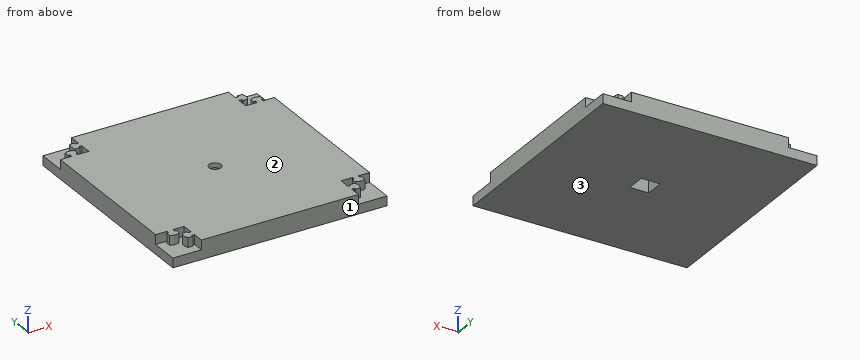
```python
from build123d import *

# Parameters (mm, degrees)
F1_DEPTH  = 40
F0_W      = 60
F0_H      = 60
F3_DEPTH  = 20
F5_DEPTH  = 20
F6_W      = 40
F6_H      = 40
F6_R      = 12.5
F7_DEPTH  = 30
F7_FACE_R = 12.5
F8_DEPTH  = 40


with BuildPart() as f1:
    # F0 (on Top) → F1 (new body)
    with BuildSketch(Plane.XY):
        Polygon((165, 165), (165, 225), (-165, 225), (-165, 165), (-225, 165), (-225, -165), (-165, -165), (-165, -225), (165, -225), (165, -165), (225, -165), (225, 165), align=None)
    extrude(amount=F1_DEPTH)

    # F0 (on Top) → F3 (join)
    with BuildSketch(Plane.XY):
        with Locations((195, 195)):
            Rectangle(F0_W, F0_H)
        Polygon((165, 165), (165, 225), (-165, 225), (-165, 165), (-225, 165), (-225, -165), (-165, -165), (-165, -225), (165, -225), (165, -165), (225, -165), (225, 165), align=None)
        with Locations((-195, 195)):
            Rectangle(F0_W, F0_H)
        with Locations((195, -195)):
            Rectangle(F0_W, F0_H)
        with Locations((-195, -195)):
            Rectangle(F0_W, F0_H)
    extrude(amount=F3_DEPTH)

    # F4 (on face) → F5 (join, through all)
    with BuildSketch(Plane.XY.offset(40)):
        with BuildLine():
            Line((-201, 171), (-201, 165))
            Line((-201, 165), (-189, 165))
            Line((-189, 165), (-189, 171))
            Line((-189, 171), (-185, 171))
            Line((-185, 171), (-185, 181))
            ThreePointArc((-185, 181), (-195, 183.679492), (-205, 181))
            Line((-205, 181), (-205, 171))
            Line((-205, 171), (-201, 171))
        make_face()
        with BuildLine():
            Line((-171, 189), (-165, 189))
            Line((-165, 189), (-165, 201))
            Line((-165, 201), (-171, 201))
            Line((-171, 201), (-171, 205))
            Line((-171, 205), (-181, 205))
            ThreePointArc((-181, 205), (-183.679492, 195), (-181, 185))
            Line((-181, 185), (-171, 185))
            Line((-171, 185), (-171, 189))
        make_face()
        with BuildLine():
            Line((181, 205), (171, 205))
            Line((171, 205), (171, 201))
            Line((171, 201), (165, 201))
            Line((165, 201), (165, 189))
            Line((165, 189), (171, 189))
            Line((171, 189), (171, 185))
            Line((171, 185), (181, 185))
            ThreePointArc((181, 185), (183.679492, 195), (181, 205))
        make_face()
        with BuildLine():
            Line((185, 181), (185, 171))
            Line((185, 171), (189, 171))
            Line((189, 171), (189, 165))
            Line((189, 165), (201, 165))
            Line((201, 165), (201, 171))
            Line((201, 171), (205, 171))
            Line((205, 171), (205, 181))
            ThreePointArc((205, 181), (195, 183.679492), (185, 181))
        make_face()
        with BuildLine():
            Line((-181, -205), (-171, -205))
            Line((-171, -205), (-171, -201))
            Line((-171, -201), (-165, -201))
            Line((-165, -201), (-165, -189))
            Line((-165, -189), (-171, -189))
            Line((-171, -189), (-171, -185))
            Line((-171, -185), (-181, -185))
            ThreePointArc((-181, -185), (-183.679492, -195), (-181, -205))
        make_face()
        with BuildLine():
            Line((-185, -181), (-185, -171))
            Line((-185, -171), (-189, -171))
            Line((-189, -171), (-189, -165))
            Line((-189, -165), (-201, -165))
            Line((-201, -165), (-201, -171))
            Line((-201, -171), (-205, -171))
            Line((-205, -171), (-205, -181))
            ThreePointArc((-205, -181), (-195, -183.679492), (-185, -181))
        make_face()
        with BuildLine():
            Line((205, -181), (205, -171))
            Line((205, -171), (201, -171))
            Line((201, -171), (201, -165))
            Line((201, -165), (189, -165))
            Line((189, -165), (189, -171))
            Line((189, -171), (185, -171))
            Line((185, -171), (185, -181))
            ThreePointArc((185, -181), (195, -183.679492), (205, -181))
        make_face()
        with BuildLine():
            Line((181, -185), (171, -185))
            Line((171, -185), (171, -189))
            Line((171, -189), (165, -189))
            Line((165, -189), (165, -201))
            Line((165, -201), (171, -201))
            Line((171, -201), (171, -205))
            Line((171, -205), (181, -205))
            ThreePointArc((181, -205), (183.679492, -195), (181, -185))
        make_face()
    extrude(amount=-F5_DEPTH)

    # F6 (on face) → F7 (cut)
    with BuildSketch(Plane(origin=(0, 0, 0), x_dir=(1, 0, 0), z_dir=(0, 0, -1))):
        Rectangle(F6_W, F6_H)
        Circle(F6_R, mode=Mode.SUBTRACT)
    extrude(amount=-F7_DEPTH, mode=Mode.SUBTRACT)

    # F7_face (on face) → F8 (cut, through all)
    with BuildSketch(Plane(origin=(0, 0, 0), x_dir=(1, 0, 0), z_dir=(0, 0, -1))):
        Circle(F7_FACE_R)
    extrude(amount=-F8_DEPTH, mode=Mode.SUBTRACT)


solid = f1.part
```
The model under review builds one solid part; all positions refer to its coordinate system, in mm. Face numbers are marked on the shaded views. Round coordinates to 2 decimals unless told otherwise and drop trailing zeros. Order: outer loops, then holes, each group sorted by start corner. A loop starts at its lowest first (then second) coordinate and runs counter-clockwise, first axis right, second up. Notation, with made-up numbers: (-36.75, -23.75) -> (8.25, -23.75) arc R21 ccw to (8.25, -7.75) -> close; hole circle Ø2 at (76, -36). An arc over 180 degrees is marked (long way). Use a Markdown table: item, result.
Q1. Clearance check with flat-ended pins moving along their axes: P1, Ø6.5, axis at y = -169, z = 27, coming from the +X side; P2, Ø6.5, axis at x = -169, z = 35, coming from the +Y side; P3, Ø1.8, axis at y = 167, z = 34, coming from the +X side. State where each tip first meets the part, or that it passes through.
Values:
| item | result |
|---|---|
| P1 | stops at x = 205 |
| P2 | stops at y = 205 |
| P3 | stops at x = 201 |
Q2. Mouldability with a two-part tool opening along Z and no side actions: class the marked faces 1, 2 and 3 as +Z half, -Z half, draft (parallel to the pull), parting line (faces both ways), or undercut.
Values:
| item | result |
|---|---|
| face 1 | draft |
| face 2 | +Z half |
| face 3 | -Z half |
Q3. We need section A-A on y = 0. Write out the cut boundary in (x, z), then the cut area to 4 significant figures.
Values:
| item | result |
|---|---|
| outline | (-225, 0) -> (-20, 0) -> (-20, 30) -> (-12.5, 30) -> (-12.5, 40) -> (-225, 40) -> close; (12.5, 30) -> (20, 30) -> (20, 0) -> (225, 0) -> (225, 40) -> (12.5, 40) -> close |
| area | 16,550 mm^2 |
Q4. For line 1 (Y direction, x = 174, z = 28.5); line 2 (X direction, y = 0, z = 38), list the stretches that pass through material, from the lowest coordinate up.
Values:
| item | result |
|---|---|
| line 1 | y = -205 to -185, -165 to 165, 185 to 205 |
| line 2 | x = -225 to -12.5, 12.5 to 225 |
